Design review of the part shown in the three views and the two pictorial views. Dimensions are in mm from the part's minimum x, y and z. Round coordinates to 2 decimals unless told otherwise and drop trailing zeros. Loops run counter-clockwise (first coordinate to the right, second up) from the corner with the lowest first, then second, coordinate; pieces in that order, holes last. Notation, with made-up numbers: M 81,4 L 92,4 A25 cw 92,31 Z; hole C 3.5,-20.75 d2. An arc over 180 degrees is marked long. One line per question, with ' | ' between items. Start each with the question number.
1) We need section C-C (y = 51.5). Give the boundary of the cut face in (x, z) (1 decimal).
2) We need section B-B (x = 188). Give the boundary of the cut face in (y, z).
3) For pin 1 Ø1.5 at (x, z) = (177.5, 20) entering from +Y; pin 2 Ø1 at (y, z) = (59.5, 84.5) entering from -X (1 decimal); pin 3 Ø1.5 at (x, z) = (184, 49.5) entering from +Y, all flat-tipped, find the tip position at first contact; note any pin that passes through.
4) For probe 1 along Y at (x, z) = (200.5, 51.5); probe 2 along Y at (x, z) = (113, 101); probe 3 along X at (y, z) = (17.5, 32) (1 decimal), list the stretches that pass through material, from the lowest coordinate up. Write a range as from..to.
5) We need section A-A (z = 72). Give the boundary of the cut face in (x, y) (1 decimal).
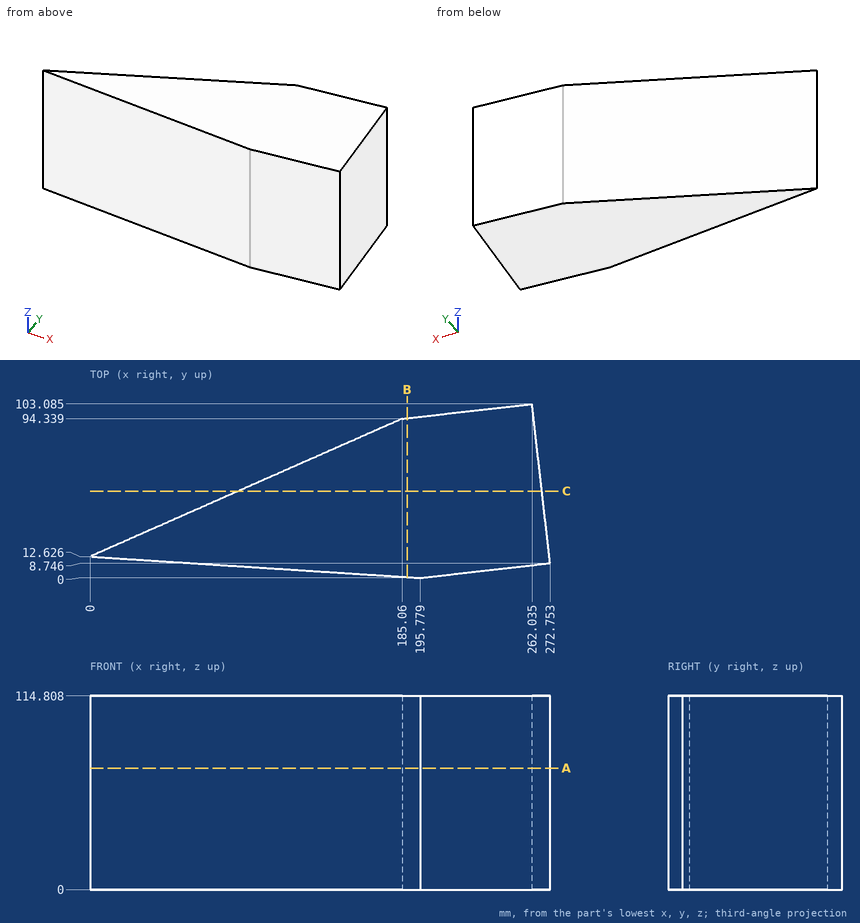
Answers below:
1) outline: M 88,0 L 267.9,0 L 267.9,114.8 L 88,114.8 Z
2) outline: M 0.5,0 L 94.67,0 L 94.67,114.81 L 0.5,114.81 Z
3) pin 1: y = 91.33 | pin 2: x = 105 | pin 3: y = 94.2
4) probe 1: 0.54..96.09 | probe 2: 5.34..62.52 | probe 3: 11..271.8
5) outline: M 0,12.6 L 195.8,0 L 272.8,8.7 L 262,103.1 L 185.1,94.3 Z
